from build123d import *

# Parameters (mm, degrees)
F0_W          = 25.4
F0_H          = 25.4
F1_DEPTH      = 5.08
F2_W          = 22.352
F2_H          = 22.352
F3_DEPTH      = 25.4
F3_DEPTH_BACK = 25.4


with BuildPart() as f1:
    # F0 (on Front) → F1 (new body)
    with BuildSketch(Plane.XZ):
        with Locations((-13.602283, -12.769573)):
            Rectangle(F0_W, F0_H)
    extrude(amount=F1_DEPTH)

    # F2 (on face) → F3 (cut, two sides)
    with BuildSketch(Plane.XZ.offset(5.08)) as f3_sk:
        with Locations((-13.602283, -12.769573)):
            Rectangle(F2_W, F2_H)
    extrude(amount=-F3_DEPTH, mode=Mode.SUBTRACT)
    extrude(f3_sk.sketch, amount=-F3_DEPTH_BACK, mode=Mode.SUBTRACT)


solid = f1.part
Geometry check sheet. Reference: the model listing, model coordinates, mm. A direction names the side the tool comes from. Give positions to 0.01 mm unless a question says otherwise; leave off trailing zeros. Loops run counter-clockwise (first coordinate to the right, second up) from the corner with the lowest first, then second, coordinate; pieces in that order, holes last.
(1) Depth check by flat-ended pin: pin 1 Ø6 at (x, z) = (-14.5, -6.5) entering from -Y; pin 2 Ø6 at (x, z) = (-22.5, -16) entering from -Y. Enter the tip coordinate at first touch or a pass-through.
From the geometry:
pin 1: passes through
pin 2: stops at y = -5.08
(2) Section check C-C on x = -19.25. Record the cut outline in (y, z), then the cut area to 3 significant figures.
From the geometry:
outline: (-5.08, -25.47) - (0, -25.47) - (0, -23.95) - (-5.08, -23.95) - close; (-5.08, -1.59) - (0, -1.59) - (0, -0.07) - (-5.08, -0.07) - close
area: 15.5 mm2
(3) Section check A-A on y = -0.8. Record the cut outline in (x, z).
From the geometry:
outline: (-26.3, -25.47) - (-0.9, -25.47) - (-0.9, -0.07) - (-26.3, -0.07) - close; hole (-24.78, -23.95) - (-2.43, -23.95) - (-2.43, -1.59) - (-24.78, -1.59) - close
(4) Set-up check for faces 1 (the flat face through (-25, -5.08, -13)), 2 (the flat face through (-2.426, -3, -13)): record each of +Z, -Z, +X, -X, +Y, -Y from which the full face is reachable in a straight line by a thin tool's end or side.
From the geometry:
face 1: +Z, -Z, +X, -X, -Y
face 2: +Y, -Y
(5) Thickness scan on L1, parallel to Z at x = -13.75, y = -1; L2, parallel to X at y = -3.45, z = -13.25. Record the ranges inside material, lowest first.
From the geometry:
L1: z = -25.47 to -23.95, -1.59 to -0.07
L2: x = -26.3 to -24.78, -2.43 to -0.9
(6) Section check B-B on z = -6.5. Record the cut outline in (x, y), then the cut area to 3 significant figures.
From the geometry:
outline: (-26.3, -5.08) - (-24.78, -5.08) - (-24.78, 0) - (-26.3, 0) - close; (-2.43, -5.08) - (-0.9, -5.08) - (-0.9, 0) - (-2.43, 0) - close
area: 15.5 mm2
(7) Release check for a two-part mould opening along X. For faces 3 (the flat face through (-14, -3, -23.946)), 4 (the flat face through (-26.302, -3, -13)), 5 (the flat face through (-25, 0, -13)) record: released by +X, released by -X, zero draft, split by the parting line, or undercut.
From the geometry:
face 3: undercut
face 4: released by -X
face 5: zero draft
